```python
from build123d import *

# Parameters (mm, degrees)
F0_R      = 12.7
F1_DEPTH  = 16.51
F2_R      = 9.398
F3_DEPTH  = 10.16
F4_R      = 5.715
F5_DEPTH  = 6.35
F6_R      = 8.001
F7_DEPTH  = 2.54
F8_R      = 7.112
F9_DEPTH  = 5.334
F10_R     = 8.001
F11_DEPTH = 15.24
F12_SIZE2 = 5.08
F12_SIZE  = 1.27
F13_R     = 5.08
F14_DEPTH = 25.4


with BuildPart() as f1:
    # F0 (on Top) → F1 (new body)
    with BuildSketch(Plane.XY):
        with Locations((-47.5551895797, -9.232012555)):
            Circle(F0_R)
    extrude(amount=-F1_DEPTH)

    # F2 (on face) → F3 (cut)
    with BuildSketch(Plane.XY):
        with Locations((-47.5551895797, -9.232012555)):
            Circle(F2_R)
    extrude(amount=-F3_DEPTH, mode=Mode.SUBTRACT)

    # F4 (on face) → F5 (cut)
    with BuildSketch(Plane.XY.offset(-10.16)):
        with Locations((-47.5551895797, -9.232012555)):
            Circle(F4_R)
    extrude(amount=-F5_DEPTH, mode=Mode.SUBTRACT)

    # F6 (on face) → F7 (join)
    with BuildSketch(Plane(origin=(0, 0, -16.51), x_dir=(1, 0, 0), z_dir=(0, 0, -1))):
        with Locations((-47.5551895797, 9.232012555)):
            Circle(F6_R)
    extrude(amount=F7_DEPTH)

    # F8 (on face) → F9 (join)
    with BuildSketch(Plane(origin=(0, 0, -19.05), x_dir=(1, 0, 0), z_dir=(0, 0, -1))):
        with Locations((-47.5551895797, 9.232012555)):
            Circle(F8_R)
    extrude(amount=F9_DEPTH)

    # F10 (on face) → F11 (join)
    with BuildSketch(Plane(origin=(0, 0, -24.384), x_dir=(1, 0, 0), z_dir=(0, 0, -1))):
        with Locations((-47.5551895797, 9.232012555)):
            Circle(F10_R)
    extrude(amount=F11_DEPTH)

    # F12
    f12_edges = [f1.edges().sort_by_distance(p)[0] for p in [
        (-55.55619, -9.232013, -39.624),
    ]]
    f12_side = f1.faces().sort_by_distance((-47.55519, -9.232013, -39.624))[0]
    chamfer(f12_edges, length=F12_SIZE, length2=F12_SIZE2, reference=f12_side)

    # F13 (on face) → F14 (cut)
    with BuildSketch(Plane(origin=(0, 0, -39.624), x_dir=(1, 0, 0), z_dir=(0, 0, -1))):
        with Locations((-47.5551895797, 9.232012555)):
            Circle(F13_R)
    extrude(amount=-F14_DEPTH, mode=Mode.SUBTRACT)


solid = f1.part
```
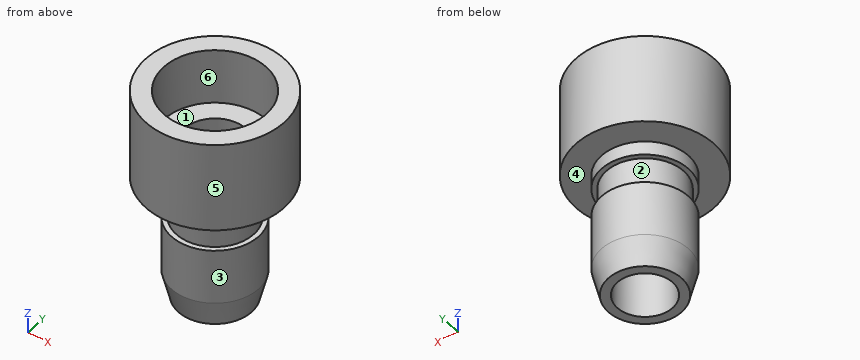
Could you check a few things on this model? Use its own coordinates, in mm. Face numbers are marked on the shaded views. A direction names the side the tool comes from. Round coordinates to 2 decimals unless told otherwise and drop trailing zeros. Loops run counter-clockwise (first coordinate to the right, second up) from the corner with the lowest first, then second, coordinate; pieces in that order, holes last. Notation, with made-up numbers: M 8,-24 L 22,-24 A7 ccw 22,-19 Z; hole C 4,5.25 d4. An arc over 180 degrees is marked long. Answer as CSV lines item,"result".
1) Imagine slicing it at C-C on y = -19.5. List the corners of the cut face in (x, z) for me, and give its area (3 significant figures).
From the geometry:
outline,"M -55.03,-16.51 L -40.08,-16.51 L -40.08,0 L -55.03,0 Z"
area,"247 mm^2"
2) Imagine slicing it at D-D on z = -14.5. List the corners of the cut face in (x, y) for me (3 decimals), and give its area (3 significant figures).
From the geometry:
outline,"C -47.555,-9.232 d25.4; hole C -47.555,-9.232 d11.43"
area,"404 mm^2"
3) Imagine slicing it at A-A on x = -39. List the corners of the cut face in (y, z) for me.
From the geometry:
outline,"M -18.62,-16.51 L 0.15,-16.51 L 0.15,0 L -5.34,0 L -5.34,-10.16 L -13.12,-10.16 L -13.12,0 L -18.62,0 Z"
4) Imagine slicing it at B-B on z = -37. List the corners of the cut face in (x, y) for me.
From the geometry:
outline,"C -47.56,-9.23 d14.77; hole C -47.56,-9.23 d10.16"
5) We'd pull the mould along X, two halves only. Please class the marked faces 4, 5 and 6: released by +X, released by -X, zero draft, split by the parting line, or undercut.
From the geometry:
face 4,"zero draft"
face 5,"split by the parting line"
face 6,"undercut"
6) Which directions (+Z, -Z, +X, -X, +Y, -Y) give clear straight access to the entire face, cutting with the end or side of a thin tool? Please do the marked faces 1, 2 and 3.
From the geometry:
face 1,"+Z"
face 2,"none"
face 3,"-Z"
7) If I drill on probe 1 along Z at (x, y) = (-35.75, -11.25); probe 2 along Z at (x, y) = (-43.5, -1.5); probe 3 along X at (y, z) = (-10.25, -7), over which ranges is the centre line in solid material (lowest first)?
From the geometry:
probe 1,"-16.51 to 0"
probe 2,"-16.51 to -10.16"
probe 3,"-60.21 to -56.9, -38.21 to -34.9"
8) For pin 1 Ø5 at (x, y) = (-57.5, -19) entering from -Z; pin 2 Ø15 at (x, y) = (-47.56, -9.23) entering from +Z; pin 3 Ø4 at (y, z) = (-16.5, -30) entering from +X, each with a flat end and sliding along its axis, tell me the tip position at first contact or that it passes through.
From the geometry:
pin 1,"z = -16.51"
pin 2,"z = -10.16"
pin 3,"x = -41.53"
